```python
from build123d import *

# Parameters (mm, degrees)
F1_R     = 31.75
F1_R_2   = 25.399999693
F3_R     = 127
F4_DEPTH = 50.8
F5_SIZE  = 3.81


with BuildPart() as f2:
    # F2: sweep along a path in F0
    with BuildLine(Plane.XY) as f2_path:
        Line((0, 0), (0, 6.35))
        ThreePointArc((0, 6.35), (13.0191035763, 37.7808964237), (44.45, 50.8))
        Line((44.45, 50.8), (50.8, 50.8))
    # F1 (on Front) → F2 (sweep)
    with BuildSketch(Plane.XZ):
        Circle(F1_R)
        Circle(F1_R_2, mode=Mode.SUBTRACT)
    sweep(path=f2_path.line)

    # F3 (on Top) → F4 (cut, symmetric)
    with BuildSketch(Plane.XY):
        with Locations((0, -122.936)):
            Circle(F3_R)
    extrude(amount=F4_DEPTH, both=True, mode=Mode.SUBTRACT)

    # F5
    f5_edges = [f2.edges().sort_by_distance(p)[0] for p in [
        (50.8, 82.55, 0),
    ]]
    chamfer(f5_edges, length=F5_SIZE)


solid = f2.part
```
Can you work these out from the model? Positions are in its coordinate system, mm. A direction names the side the tool comes from. Give positions to 0.01 mm unless a question says otherwise; leave off trailing zeros. Loops run counter-clockwise (first coordinate to the right, second up) from the corner with the lowest first, then second, coordinate; pieces in that order, holes last. Notation, with made-up numbers: M -17.5,-29 L -3.5,-29 A23 cw -3.5,-7 Z; hole C 78,-22.5 d4. An arc over 180 degrees is marked long. Use one line per item in the form item = value. Start each with the question number.
(1) Please list where these lines run through material, in increasing order: line 1 (X direction, y = 3.4, z = 0); line 2 (Y direction, x = 47, z = 0); line 3 (Z direction, x = 44, y = 50).
(2) Thinking about a two-plate mould opening in Y: for faces 1 (the cylindrical face through (2.53, 4.04, -25.93)), 2 (the flat face through (50.8, 76, -6)), 3 (the cylindrical face through (47.669, 27.337, 9.728)), which applies, released by +Y, released by -Y, zero draft, split by the parting line, or undercut?
(3) On a 3-axis mill with a long thin cutter (end or side, diameter ignored), from which of +Z, -Z, +X, -X, +Y, -Y can I reach the whole of each face in a straight line? I mean faces 4 (the cylindrical face through (14.65, 3.94, 28.17)), 5 (the cylindrical face through (45.74, 82.52, -1.4)). Say none if no direction works.
(4) I want a section at A-A, the plane z = 0. Write out the boundary of the cut face in (x, y).
(5) I'm going to push flat-ended pins straight in: P1, Ø2, axis at x = 5.5, z = 8.5, coming from the +Y side; P2, Ø2, axis at x = -21, y = 18, coming from the +Z side; P3, Ø8, axis at x = 33, y = 58, coming from the +Z side. Where does each tip first touch, or does it pass through?
Worked out:
q1.line_1 = -31.75 to -25.4, 25.4 to 31.75
q1.line_2 = 19.06 to 25.4, 76.2 to 82.54
q1.line_3 = -31.74 to -25.39, 25.39 to 31.74
q2.face_1 = released by -Y
q2.face_2 = zero draft
q2.face_3 = undercut
q3.face_4 = -Y
q3.face_5 = +X
q4.outline = M -31.75,0.03 A127 cw -25.4,1.5 L -25.4,6.35 A69.85 cw 44.45,76.2 L 50.8,76.2 L 50.8,78.74 L 46.99,82.55 L 44.45,82.55 A76.2 ccw -31.75,6.35 Z; M 25.4,1.5 A127 cw 31.75,0.03 L 31.75,6.35 A12.7 cw 44.45,19.05 L 46.99,19.05 L 50.8,22.86 L 50.8,25.4 L 44.45,25.4 A19.05 ccw 25.4,6.35 Z
q5.P1 = 71.17
q5.P2 = 23.79
q5.P3 = 31.44
